Could you check a few things on this drawing? It's one solid part, dimensions in mm from its lowest x, y, z. A direction names the side the tool comes from. Give positions to 0.01 mm unless a question says otherwise; leave off trailing zeros. Loops run counter-clockwise (first coordinate to the right, second up) from the corner with the lowest first, then second, coordinate; pieces in that order, holes last.
1. For the marked faces 4 and 5, which set-ups out of +Z, -Z, +X, -X, +Y, -Y let a thin tool reach every point of the face, with its end or its side?
2. For P1, Ø3.5, axis at x = 1.5, y = 16.5, coming from the -Z side; P2, Ø1, axis at x = 38, z = 22.5, coming from the +Y side; P3, Ø3.5, axis at x = 50, y = 25.5, coming from the +Z side, each with a flat end and sliding along its axis, tell me the tip position at first contact or that it passes through.
3. Imagine slicing it at D-D (z = 4). List the corners of the cut face in (x, y) for me.
4. Imagine slicing it at A-A (x = 25.5). List the corners of the cut face in (y, z) for me, plus the area to 3 significant figures.
5. Imagine slicing it at B-B (y = 17). List the corners of the cut face in (x, z) for me, plus the area to 3 significant figures.
6. Thinking about a two-plate mould opening in X: for the marked faces 1, 2 and 3, which applies, +X half, -X half, draft (parallel to the pull), parting line (faces both ways), or undercut?
7. I need wall thicknesses on line 1 along Z through (x, y) = (25.5, 1.5); line 2 along X through (y, z) = (30.5, 4.5); line 3 along X through (y, z) = (3.75, 16). Which ranges of each line are inside material? Lowest first, please.
8. Imagine slicing it at C-C (z = 16). List the corners of the cut face in (x, y) for me, plus the area to 3 significant figures.
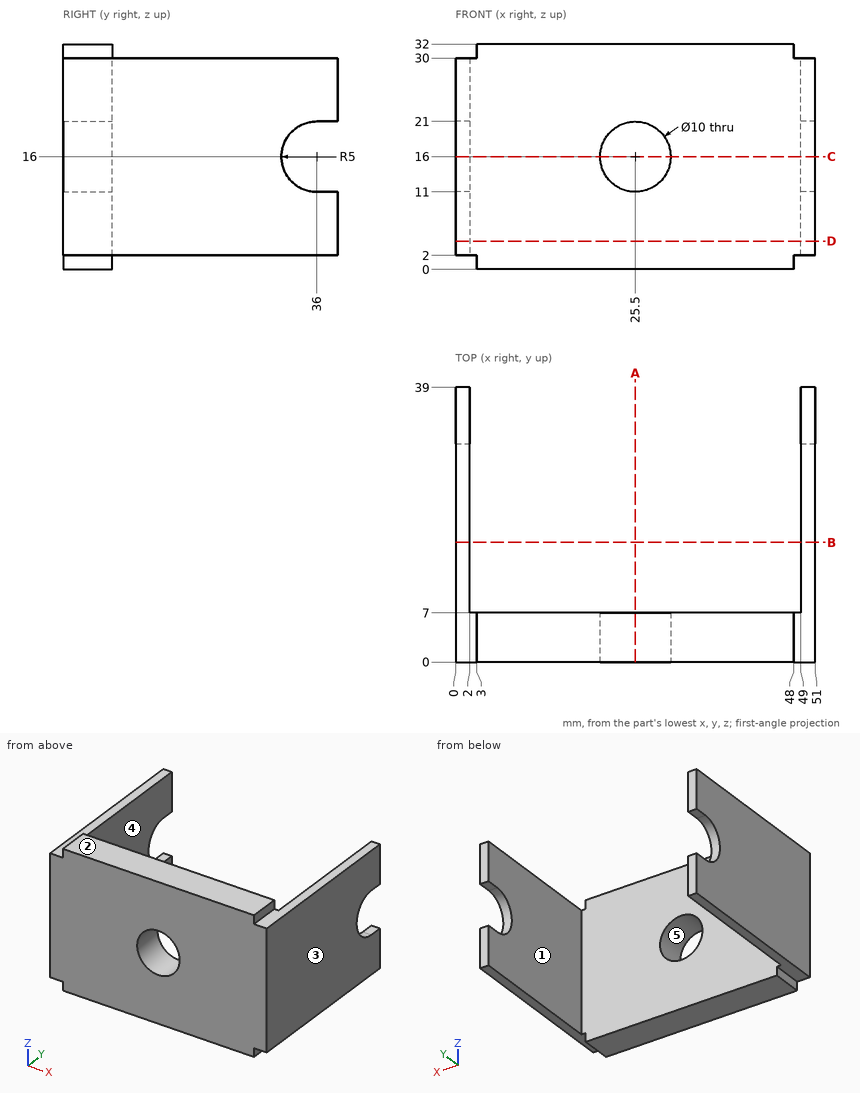
Derived:
1. face 4: +Z, -Z, +Y
1. face 5: +Y, -Y
2. P1: stops at z = 2
2. P2: stops at y = 7
2. P3: stops at z = 30
3. outline: (0, 0) - (51, 0) - (51, 39) - (49, 39) - (49, 7) - (2, 7) - (2, 39) - (0, 39) - close
4. outline: (0, 0) - (7, 0) - (7, 11) - (0, 11) - close; (0, 21) - (7, 21) - (7, 32) - (0, 32) - close
4. area: 154 mm2
5. outline: (0, 2) - (2, 2) - (2, 30) - (0, 30) - close; (49, 2) - (51, 2) - (51, 30) - (49, 30) - close
5. area: 112 mm2
6. face 1: undercut
6. face 2: draft
6. face 3: +X half
7. line 1: z = 0 to 11, 21 to 32
7. line 2: x = 0 to 2, 49 to 51
7. line 3: x = 0 to 20.5, 30.5 to 51
8. outline: (0, 0) - (20.5, 0) - (20.5, 7) - (2, 7) - (2, 31) - (0, 31) - close; (30.5, 0) - (51, 0) - (51, 31) - (49, 31) - (49, 7) - (30.5, 7) - close
8. area: 383 mm2
